```python
from build123d import *

# Parameters (mm, degrees)
F0_R        = 1.0922
F1_DEPTH    = 1.016
F2_R        = 0.3429
F3_DEPTH    = 8.382
F4_W        = 27.305
F4_H        = 19.05
F5_DEPTH    = 1.3716
F6_W        = 12.7
F6_H        = 3.8608
F7_DEPTH    = 1.3716
F8_T1_DEPTH = 34.2391400943


# Not quite as in the source:
# - a fillet or chamfer that OpenCascade refuses, or shapes differently, is made with other operations: its cross-section is extruded or revolved along the edge and cut away or added


with BuildPart() as f1:
    # F0 (on Front) → F1 (new body)
    with BuildSketch(Plane.XZ):
        with BuildLine():
            Line((11.1125, 13.6525), (-11.1125, 13.6525))
            ThreePointArc((-11.1125, 13.6525), (-12.9085512242, 12.9085512242), (-13.6525, 11.1125))
            Line((-13.6525, 11.1125), (-13.6525, -11.1125))
            ThreePointArc((-13.6525, -11.1125), (-12.9085512242, -12.9085512242), (-11.1125, -13.6525))
            Line((-11.1125, -13.6525), (11.1125, -13.6525))
            ThreePointArc((11.1125, -13.6525), (12.9085512242, -12.9085512242), (13.6525, -11.1125))
            Line((13.6525, -11.1125), (13.6525, 11.1125))
            ThreePointArc((13.6525, 11.1125), (12.9085512242, 12.9085512242), (11.1125, 13.6525))
        make_face()
        with Locations((-11.1125, -11.1125)):
            Circle(F0_R, mode=Mode.SUBTRACT)
        with Locations((11.1125, -11.1125)):
            Circle(F0_R, mode=Mode.SUBTRACT)
        with Locations((-11.1125, 11.1125)):
            Circle(F0_R, mode=Mode.SUBTRACT)
        with Locations((11.1125, 11.1125)):
            Circle(F0_R, mode=Mode.SUBTRACT)
    extrude(amount=F1_DEPTH)

    # F2 (on face) → F3 (join)
    with BuildSketch(Plane.XZ.offset(1.016)):
        with Locations((-3.81, 11.1125)):
            Circle(F2_R)
        with Locations((-1.27, 11.1125)):
            Circle(F2_R)
        with Locations((3.81, 11.1125)):
            Circle(F2_R)
        with Locations((1.27, 11.1125)):
            Circle(F2_R)
    extrude(amount=F3_DEPTH)

    # F4 (on face) → F5 (join)
    with BuildSketch(Plane(origin=(0, 0, 0), x_dir=(-1, 0, 0), z_dir=(0, 1, 0))):
        with Locations((0, -0.2667)):
            Rectangle(F4_W, F4_H)
    extrude(amount=F5_DEPTH)

    # F6 (on face) → F7 (join, through all)
    with BuildSketch(Plane(origin=(0, 0, 0), x_dir=(-1, 0, 0), z_dir=(0, 1, 0))):
        with Locations((0.0635, -11.7221)):
            Rectangle(F6_W, F6_H)
    extrude(amount=F7_DEPTH)

    # F8: fillet of radius 5.08 on 1 edges, made by hand

    # F8_s2 → F8_t1 (cut)
    with BuildSketch(Plane.YZ.offset(-17.1830700471)):
        with BuildLine():
            ThreePointArc((1.3716, -9.3446719811), (0.7347853439, -11.8072933487), (-1.016, -13.6525))
            Line((-1.016, -13.6525), (1.3716, -13.6525))
            Line((1.3716, -13.6525), (1.3716, -9.3446719811))
        make_face()
    extrude(amount=F8_T1_DEPTH, mode=Mode.SUBTRACT)


solid = f1.part
```
The listing builds one solid part. Answer for the finished solid, in the listing's coordinates (mm). A direction names the side the tool comes from. Round coordinates to 2 decimals unless told otherwise and drop trailing zeros. Loops run counter-clockwise (first coordinate to the right, second up) from the corner with the lowest first, then second, coordinate; pieces in that order, holes last. Notation, with made-up numbers: (-31.75, -34.75) - (-2.75, -34.75) arc R25 cw to (-2.75, -3.75) - close; hole circle Ø6 at (14.5, 72). An arc over 180 degrees is marked (long way). Use one line per item in the form item = value. Start each with the question number.
1. The part is cut by section B-B on y = -7. Determine the outline of the cut face in (x, z), then the cut area to 3 significant figures.
2. A tool of negligible diameter and unlimited length cuts with its end or side. For faces 1 (the face through (10, 1, -9.792)), 2 (the face through (10.31, -0.5, -10.37)), 3 (the face through (-10, 1, -9.792)), from which of +Z, -Z, +X, -X, +Y, -Y can it reach the whole face along a straight path? Write none if from no direction.
3. For a pull along X with two mould halves and no side action, classify faces 4 (the face through (-12.889, -0.501, 12.928)), 5 (the face through (6.286, 0.5, -11)), 6 (the face through (10.246, -0.501, 10.448)), 7 (the face through (0, 1.372, 0)) as pulls with the +X half, pulls with the -X half, needs draft (parallel to the pull), parting line crosses it, or undercut.
4. Consider line 1 (X direction, y = 0.25, z = -10); line 2 (Y direction, x = -4.25, z = 3.25); line 3 (Y direction, x = 4, z = 10.75). Determine where each line is inside the solid, lowest interval first. Write a range as [from, to].
5. The part is cut by section C-C on x = 3.81. Determine the outline of the cut face in (y, z), then the cut area to 3 significant figures.
6. The part is cut by section A-A on x = 11.5. Determine the outline of the cut face in (y, z).
7. Given pin 1 Ø0.9 at (x, z) = (9.5, -11.5) entering from +Y; pin 2 Ø1 at (x, y) = (10, -2) entering from -Z; pin 3 Ø13.5 at (x, z) = (0.5, -1.5) entering from -Y; pin 4 Ø1.5 at (y, z) = (-4, 10.5) entering from +X, each flat-ended and moving along its own axis, determine where each tip first touches the part or whether it passes through.
8. The part is cut by section D-D on z = 4.5. Determine the outline of the cut face in (x, y), then the cut area to 3 significant figures.
Geometry check:
q1.outline = circle Ø0.69 at (-3.81, 11.11); circle Ø0.69 at (-1.27, 11.11); circle Ø0.69 at (1.27, 11.11); circle Ø0.69 at (3.81, 11.11)
q1.area = 1.48 mm^2
q2.face_1 = -Z, +X, +Y
q2.face_2 = +Y, -Y
q2.face_3 = -Z, -X, +Y
q3.face_4 = pulls with the -X half
q3.face_5 = pulls with the +X half
q3.face_6 = undercut
q3.face_7 = needs draft
q4.line_1 = [-6.41, 6.29]
q4.line_2 = [-1.02, 1.37]
q4.line_3 = [-1.02, 0]
q5.outline = (-9.4, 10.77) - (-1.02, 10.77) - (-1.02, -13.65) arc R5.08 ccw to (1.37, -9.34) - (1.37, 9.26) - (0, 9.26) - (0, 13.65) - (-1.02, 13.65) - (-1.02, 11.46) - (-9.4, 11.46) - close
q5.area = 61.9 mm^2
q6.outline = (-1.02, -13.62) - (-0.97, -13.62) arc R5.08 ccw to (0, -12.82) - (0, -12.13) - (-1.02, -12.13) - close; (-1.02, -10.09) - (0, -10.09) - (0, -9.79) - (1.35, -9.79) arc R5.08 ccw to (1.37, -9.34) - (1.37, 9.26) - (0, 9.26) - (0, 10.09) - (-1.02, 10.09) - close; (-1.02, 12.13) - (0, 12.13) - (0, 13.62) - (-1.02, 13.62) - close
q7.pin_1 = 0
q7.pin_2 = through
q7.pin_3 = -1.02
q7.pin_4 = 4.15
q8.outline = (-13.65, -1.02) - (13.65, -1.02) - (13.65, 1.37) - (-13.65, 1.37) - close
q8.area = 65.2 mm^2
